Input: part model. Units: mm. Frame: model coordinates. Face numbers are marked on the shaded views. A direction names the side the tool comes from. Coordinates: 2 decimals unless noted, no trailing zeros. Write each loop counter-clockwise with the first axis right and the second up, starting at its lowest first coordinate (ties: lowest second). Pieces come first, ordered by that corner, then holes. Notation, with made-up numbers: (-14, -10) - (13, -10) arc R18 ccw to (13, 3) - close; hole circle Ø11 at (24, 71.5). An arc over 180 degrees is marked (long way). Use a Markdown table: item, result. Add a question column.
Q1. Set-up query: the marked faces 1, 2, 3, 4 and 5. Return all of +Z, -Z, +X, -X, +Y, -Y with unobstructed straight access to the full face (end or side cutting, diameter ignored); none if empty.
Q2. Material intervals for probe 1 along Z at (x, y) = (-30, 30) (3 decimals); probe 2 along X at (y, z) = (20.5, 4) (3 decimals); probe 3 along Y at (x, z) = (26, 14), sorted ascending. Write a range as from..to.
Q3. Pin query (flat end, axial travel): P1, Ø6, axis at y = 23.5, z = 53, coming from the -X side; P2, Ø15.5, axis at x = 67.5, z = 40, coming from the +Y side; P3, Ø8.5, axis at y = -14, z = 15.5, coming from the -X side (3 decimals). Return the tip coordinate at first contact, or that it passes through.
Q4. Section query A-A (y = 31). Return the cut outline in (x, z) (3 decimals), then the cut area to 3 significant figures.
from build123d import *

# Parameters (mm, degrees)
F1_DEPTH = 63.5
F0_W     = 27.3727922164
F0_H     = 19.05
F2_DEPTH = 25.4
F3_DEPTH = 7.9375
F5_R     = 5.08


with BuildPart() as f1:
    # F0 (on Front) → F1 (new body, symmetric)
    with BuildSketch(Plane.XZ):
        Polygon((22.225, 9.525), (-41.275, 9.525), (-41.275, -9.525), (41.275, -9.525), (41.275, 9.525), align=None)
    extrude(amount=F1_DEPTH, both=True)

    # F0 (on Front) → F2 (join, symmetric)
    with BuildSketch(Plane.XZ):
        with Locations((73.4864038918, 52.4002)):
            Rectangle(F0_W, F0_H)
        with BuildLine():
            Line((22.225, 27.0002), (22.225, 9.525))
            Line((22.225, 9.525), (41.275, 9.525))
            Line((41.275, 9.525), (41.275, 27.0002))
            ThreePointArc((41.275, 27.0002), (45.9246798487, 38.2255201513), (57.15, 42.8752))
            Line((57.15, 42.8752), (59.8000077836, 42.8752))
            Line((59.8000077836, 42.8752), (59.8000077836, 61.9252))
            Line((59.8000077836, 61.9252), (57.15, 61.9252))
            add(Edge.make_bspline(
                [(52.6023702137, 61.6278578522), (54.0985072201, 61.7416652267), (55.6143415744, 61.8409632906), (57.15, 61.9252)],
                knots=[109.0172906115, 109.0172906115, 109.0172906115, 109.0172906115, 111.5045361635, 111.5045361635, 111.5045361635, 111.5045361635], degree=3))
            ThreePointArc((52.6023702137, 61.6278578522), (30.8956518336, 50.032022059), (22.225, 27.0002))
        make_face()
    extrude(amount=F2_DEPTH, both=True)

    # F0 (on Front) → F3 (join, symmetric)
    with BuildSketch(Plane.XZ):
        with BuildLine():
            add(Edge.make_bspline(
                [(-41.275, 9.525), (-40.7097081479, 23.7773233991), (-12.9741076271, 56.6396203166), (52.6023702137, 61.6278578522)],
                knots=[0, 0, 0, 0, 109.0172906115, 109.0172906115, 109.0172906115, 109.0172906115], degree=3))
            Line((-41.275, 9.525), (22.225, 9.525))
            Line((22.225, 9.525), (22.225, 27.0002))
            ThreePointArc((22.225, 27.0002), (30.8956518336, 50.032022059), (52.6023702137, 61.6278578522))
        make_face()
    extrude(amount=F3_DEPTH, both=True)

    # F0 (on Front) → F4 (revolve)
    with BuildSketch(Plane.XZ):
        Polygon((87.1728, 66.675), (87.1728, 61.9252), (87.1728, 42.8752), (87.1728, 38.1), (110.6000077836, 38.1), (110.6000077836, 66.675), align=None)
    revolve(axis=Axis((87.1728, 0, 52.3875), (0, 0, -1)))

    # F5
    f5_edges = [f1.edges().sort_by_distance(p)[0] for p in [
        (-41.275, -63.5, 0),
        (41.275, -63.5, 0),
        (41.275, 63.5, 0),
        (-41.275, 63.5, 0),
    ]]
    fillet(f5_edges, radius=F5_R)


solid = f1.part
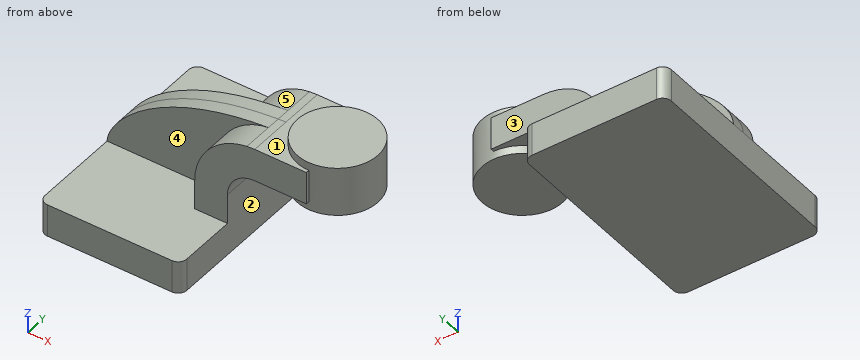
Values follow:
| question | item | result |
|---|---|---|
| 1 | face 1 | +Z, -X |
| 1 | face 2 | -Z, +X, +Y, -Y |
| 1 | face 3 | +Z, +X, -X, +Y |
| 1 | face 4 | +Z, -X, -Y |
| 1 | face 5 | +Z, -X, +Y |
| 2 | probe 1 | -9.525..9.525 |
| 2 | probe 2 | -41.275..41.275 |
| 2 | probe 3 | -25.4..25.4 |
| 3 | P1 | x = 30.87 |
| 3 | P2 | y = 25.4 |
| 3 | P3 | x = 22.225 |
| 4 | outline | (-41.275, -9.525) - (41.275, -9.525) - (41.275, 9.525) - (-41.275, 9.525) - close |
| 4 | area | 1,570 mm2 |
